from build123d import *

# Parameters (mm, degrees)
CYLINDER014005848_R     = 2.7
CYLINDER014005848_DEPTH = 3
CYLINDER014005847_R     = 4
CYLINDER014005847_DEPTH = 2


with BuildPart() as obj1:
    # Cylinder014005848 → Cylinder014005848 (new body)
    with BuildSketch(Plane.XY.offset(-1)):
        Circle(CYLINDER014005848_R)
    extrude(amount=CYLINDER014005848_DEPTH)


with BuildPart() as obj2:
    # Cylinder014005847 → Cylinder014005847 (new body)
    with BuildSketch(Plane.XY.offset(-1)):
        Circle(CYLINDER014005847_R)
    extrude(amount=CYLINDER014005847_DEPTH)

    # Cut061311: cut obj1
    add(obj1.part, mode=Mode.SUBTRACT)


solid = obj2.part
Could you check a few things on this model? Use its own coordinates, in mm. Give positions to 0.01 mm unless a question says otherwise; leave off trailing zeros. Loops run counter-clockwise (first coordinate to the right, second up) from the corner with the lowest first, then second, coordinate; pieces in that order, holes last. Notation, with made-up numbers: (85, -23) -> (141, -23) arc R28 cw to (141, 0) -> close; hole circle Ø6 at (67.5, 77.5). An arc over 180 degrees is marked (long way). Return JSON: item names as keys, results as strings.
Item 1: We'd pull the mould along Y, two halves only. Please class faces 1 (the cylindrical face through (-0.585, -2.636, -0.014)), 2 (the cylindrical face through (-0.867, -3.905, -0.014)), 3 (the flat face through (3, -1, -1)): +Y half, -Y half, draft (parallel to the pull), parting line (faces both ways), or undercut.
Geometry results:
{"face 1": "undercut", "face 2": "parting line", "face 3": "draft"}
Item 2: If we section it at C-C on z = 0.3: List the corners of the cut face in (x, y) for me, plus the area to 3 significant figures.
Geometry results:
{"outline": "circle Ø8 at (0, 0); hole circle Ø5.4 at (0, 0)", "area": "27.4 mm²"}
Item 3: I need wall thicknesses on L1, parallel to Y at x = 0, z = 0.4; L2, parallel to Y at x = -1.25, z = 0. Which ranges of each line are inside material? Lowest first, please. Write a range as from..to.
Geometry results:
{"L1": "y = -4..-2.7, 2.7..4", "L2": "y = -3.8..-2.39, 2.39..3.8"}
Item 4: If we section it at D-D on x = 3.25: List the corners of the cut face in (y, z) for me, plus the area to 3 significant figures.
Geometry results:
{"outline": "(-2.33, -1) -> (2.33, -1) -> (2.33, 1) -> (-2.33, 1) -> close", "area": "9.33 mm²"}
Item 5: If we section it at A-A on x = 0: List the corners of the cut face in (y, z) for me.
Geometry results:
{"outline": "(-4, -1) -> (-2.7, -1) -> (-2.7, 1) -> (-4, 1) -> close; (2.7, -1) -> (4, -1) -> (4, 1) -> (2.7, 1) -> close"}
